Here's the drawing with two shaded views (mm, measured from the low corner). I have some questions. A direction names the side the tool comes from. Coordinates: 2 decimals unless noted, no trailing zeros. Write each loop counter-clockwise with the first axis right and the second up, starting at its lowest first coordinate (ties: lowest second). Pieces come first, ordered by that corner, then holes. Notation, with made-up numbers: (16.25, -7) -> (45.25, -7) arc R19 ccw to (45.25, 23) -> close; hole circle Ø7 at (25, -24.75). An arc over 180 degrees is marked (long way). Use a Markdown table: item, result. Add a question column.
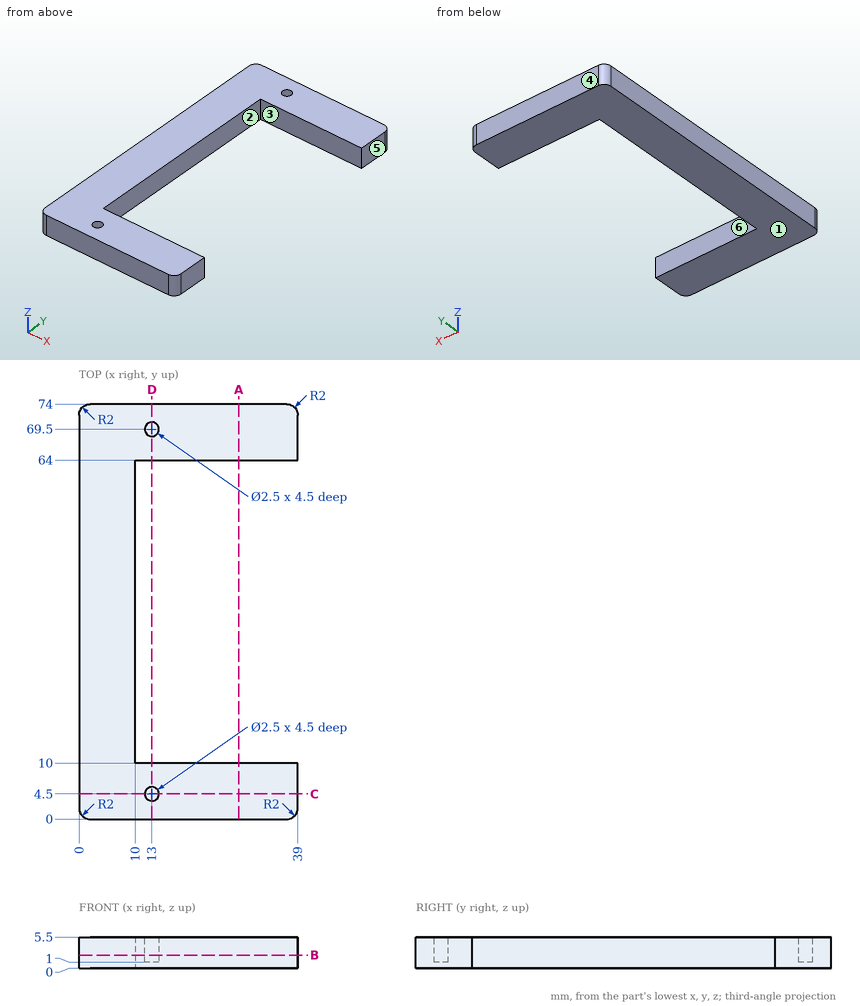
Q1. Which directions (+Z, -Z, +X, -X, +Y, -Y) give clear straight access to the entire face, cutting with the end or side of a thin tool? Please do the marked faces 1 and 2.
Q2. Suppose I cut it at B-B, the plane z = 2.3. Write out the boundary of the cut face in (x, y), and give its area (3 significant figures).
Q3. Suppose I cut it at D-D, the plane x = 13. Write out the boundary of the cut face in (y, z).
Q4. Suppose I cut it at A-A, the plane x = 28.5. Write out the boundary of the cut face in (y, z).
Q5. Will these pins go through, and if not, where does the flat tip stop? pin 1 (2 mm diameter, centred on y = 38, z = 2.5, fed in from +X); pin 2 (1.2 mm diameter, centred on x = 13, y = 69, fed in from +Z).
Q6. Suppose I cut it at C-C, the plane y = 4.5. Write out the boundary of the cut face in (x, z), and give its area (3 significant figures).
Q7. Please list where these lines run through material, in increasing order: line 1 (Y direction, x = 13, z = 2.7); line 2 (Y direction, x = 37, z = 0.85); line 3 (X direction, y = 69.5, z = 2.35).
Q8. Thinking about a two-plate mould opening in Y: for the marked faces 3, 4, 5 and 6, which applies, released by +Y, released by -Y, zero draft, split by the parting line, or undercut?
Answer key:
| question | item | result |
|---|---|---|
| 1 | face 1 | -Z, +X, -X, +Y, -Y |
| 1 | face 2 | +Z, -Z, +X |
| 2 | outline | (0, 2) arc R2 ccw to (2, 0) -> (37, 0) arc R2 ccw to (39, 2) -> (39, 10) -> (10, 10) -> (10, 64) -> (39, 64) -> (39, 72) arc R2 ccw to (37, 74) -> (2, 74) arc R2 ccw to (0, 72) -> close; hole circle Ø2.5 at (13, 4.5); hole circle Ø2.5 at (13, 69.5) |
| 2 | area | 1,310 mm^2 |
| 3 | outline | (0, 0) -> (10, 0) -> (10, 5.5) -> (5.75, 5.5) -> (5.75, 1) -> (3.25, 1) -> (3.25, 5.5) -> (0, 5.5) -> close; (64, 0) -> (74, 0) -> (74, 5.5) -> (70.75, 5.5) -> (70.75, 1) -> (68.25, 1) -> (68.25, 5.5) -> (64, 5.5) -> close |
| 4 | outline | (0, 0) -> (10, 0) -> (10, 5.5) -> (0, 5.5) -> close; (64, 0) -> (74, 0) -> (74, 5.5) -> (64, 5.5) -> close |
| 5 | pin 1 | stops at x = 10 |
| 5 | pin 2 | stops at z = 1 |
| 6 | outline | (0, 0) -> (39, 0) -> (39, 5.5) -> (14.25, 5.5) -> (14.25, 1) -> (11.75, 1) -> (11.75, 5.5) -> (0, 5.5) -> close |
| 6 | area | 203 mm^2 |
| 7 | line 1 | y = 0 to 3.25, 5.75 to 10, 64 to 68.25, 70.75 to 74 |
| 7 | line 2 | y = 0 to 10, 64 to 74 |
| 7 | line 3 | x = 0 to 11.75, 14.25 to 39 |
| 8 | face 3 | undercut |
| 8 | face 4 | released by +Y |
| 8 | face 5 | zero draft |
| 8 | face 6 | undercut |
